The listing builds one solid part. Answer for the finished solid, in the listing's coordinates (mm). Face numbers are marked on the shaded views. A direction names the side the tool comes from. Give positions to 0.01 mm unless a question says otherwise; leave off trailing zeros. Loops run counter-clockwise (first coordinate to the right, second up) from the corner with the lowest first, then second, coordinate; pieces in that order, holes last. Notation, with made-up numbers: (46.5, 64) - (105.5, 64) arc R24 ccw to (105.5, 98) - close; hole circle Ø6 at (46.25, 43). An arc over 180 degrees is marked (long way). Write item = value, one per line. Start each with the question number.
1) The part is cut by section B-B on z = 15. Write down the section's boundary in (x, y).
2) Flat-ended cylindrical pins translate along their axes: P1, Ø11, axis at y = 73.5, z = 65, coming from the +X side; P2, Ø18, axis at x = 263, z = 30.5, coming from the -Y side. Find the tip coordinate at first contact, or state that the pin passes through.
3) Consider probe 1 along Y at (x, z) = (166, 4); probe 2 along X at (y, z) = (36.5, 35). Determine where each line is inside the solid, lowest interval first.
4) Which of the six approach directions +Z, -Z, +X, -X, +Y, -Y give full straight-line access (tool end or side, diameter ignored) to the marked faces 1 and 2?
5) The part is cut by section A-A on x = 342.5. Write down the section's boundary in (y, z), plus the area to 3 significant figures.
from build123d import *

# Parameters (mm, degrees)
EXTRUDE_1_DEPTH     = 70
SKETCH_3_W          = 10
SKETCH_3_H          = 10
CUT_EXTRUDE_1_DEPTH = 210
SKETCH_4_W          = 10
SKETCH_4_H          = 10
CUT_EXTRUDE_2_DEPTH = 340


with BuildPart() as part:
    # Эскиз2 → Бобышка-Вытянуть1 (new body)
    with BuildSketch(Plane.XY):
        Polygon((0, 0), (0, 250), (400, 250), (400, 200), (60, 200), (60, 0), align=None)
    extrude(amount=EXTRUDE_1_DEPTH)

    # Эскиз3 → Вырез-Вытянуть1 (cut)
    with BuildSketch(Plane.XZ):
        with Locations((55, 65)):
            Rectangle(SKETCH_3_W, SKETCH_3_H)
    extrude(amount=-CUT_EXTRUDE_1_DEPTH, mode=Mode.SUBTRACT)

    # Эскиз4 → Вырез-Вытянуть2 (cut)
    with BuildSketch(Plane(origin=(400, 0, 0), x_dir=(0, 0, -1), z_dir=(1, 0, 0))):
        with Locations((-65, 205)):
            Rectangle(SKETCH_4_W, SKETCH_4_H)
    extrude(amount=-CUT_EXTRUDE_2_DEPTH, mode=Mode.SUBTRACT)


solid = part.part
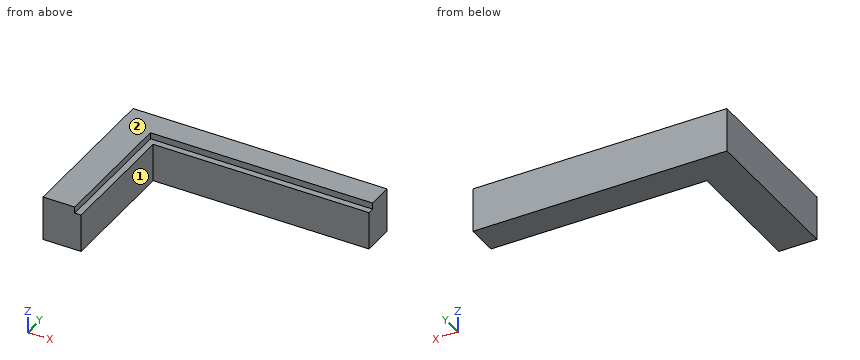
Answer below:
q1.outline = (0, 0) - (60, 0) - (60, 200) - (400, 200) - (400, 250) - (0, 250) - close
q2.P1 = 60
q2.P2 = 200
q3.probe_1 = 200 to 250
q3.probe_2 = 0 to 60
q4.face_1 = +Z, -Z, +X, -Y
q4.face_2 = +Z, +X, -X, +Y, -Y
q5.outline = (200, 0) - (250, 0) - (250, 70) - (210, 70) - (210, 60) - (200, 60) - close
q5.area = 3,400 mm2
